The listing builds one solid part. Answer for the finished solid, in the listing's coordinates (mm). Coordinates: 2 decimals unless noted, no trailing zeros. Order: outer loops, then holes, each group sorted by start corner. A loop starts at its lowest first (then second) coordinate and runs counter-clockwise, first axis right, second up. Notation, with made-up numbers: (-22, 10.5) -> (17, 10.5) arc R31 cw to (17, 48.5) -> close; hole circle Ø10 at (20, 10.25). An arc over 180 degrees is marked (long way). Write item = value, one per line. Start each with the question number.
```python
from build123d import *

# Parameters (mm, degrees)
SKETCH3_R                = 76.2
BOSS_EXTRUDE1_DEPTH      = 6.35
BOSS_EXTRUDE1_DEPTH_BACK = 6.35
SKETCH4_R                = 13.0175
SKETCH4_R_2              = 5.953125
CUT_EXTRUDE1_DEPTH       = 13.7


with BuildPart() as part:
    # Sketch3 → Boss-Extrude1 (new body, two sides)
    with BuildSketch(Plane(origin=(0, 0, 0), x_dir=(1, 0, 0), z_dir=(0, 1, 0))) as boss_extrude1_sk:
        Circle(SKETCH3_R)
    extrude(amount=BOSS_EXTRUDE1_DEPTH)
    extrude(boss_extrude1_sk.sketch, amount=-BOSS_EXTRUDE1_DEPTH_BACK)

    # Sketch4 → Cut-Extrude1 (cut, through all)
    with BuildSketch(Plane(origin=(0, 6.35, 0), x_dir=(1, 0, 0), z_dir=(0, 1, 0))):
        Circle(SKETCH4_R)
        with Locations((0, 57.15)):
            Circle(SKETCH4_R_2)
        with Locations((49.493351826, -28.575)):
            Circle(SKETCH4_R_2)
        with Locations((-49.493351826, -28.575)):
            Circle(SKETCH4_R_2)
    extrude(amount=-CUT_EXTRUDE1_DEPTH, mode=Mode.SUBTRACT)


solid = part.part
```
Item 1: Each of these flat-tipped pins is pushed along its axis until it touches: pin 1 (2 mm diameter, centred on y = 2.5, z = 22.5, fed in from +X); pin 2 (15.5 mm diameter, centred on x = 0, z = 0, fed in from -Y); pin 3 (5 mm diameter, centred on x = 10, y = 4.5, fed in from -Z); pin 4 (3 mm diameter, centred on y = 1.5, z = -41.5, fed in from +X). Where does it stop, or does it pass through?
Item 2: Section D-D, the plane z = -57.15 is taken. Give the vertices of the cut face in (x, y), then the cut area to 3 significant figures.
Item 3: For a pull along Z with two mould halves and no side action, classify faces 1 (the flat face through (16, -6.35, -1)), 2 (the cylindrical face through (-46.75, 0.09, 33.86)), 3 (the cylindrical face through (-60.47, 0.089, 46.367)) as pulls with the +Z half, pulls with the -Z half, needs draft (parallel to the pull), parting line crosses it, or undercut.
Item 4: Section C-C, the plane y = 1.5 is taken. Give the number of separate pieces and of enclosed holes in the cut face, then the cut area to 3 significant figures.
Item 5: Consider probe 1 along Z at (x, y) = (0, -1.25); probe 2 along X at (y, z) = (-4, 27); probe 3 along X at (y, z) = (4.75, -53). Determine where each line is inside the solid, lowest interval first.
Item 6: Section A-A, the plane z = 0 is taken. Give the vertices of the cut face in (x, y).
Item 7: Section B-B, the plane x = 0 is taken. Give the vertices of the cut face in (y, z), then the cut area to 3 significant figures.
A:
q1.pin_1 = 73.1
q1.pin_2 = through
q1.pin_3 = -75.83
q1.pin_4 = 64.86
q2.outline = (-50.4, -6.35) -> (-5.95, -6.35) -> (-5.95, 6.35) -> (-50.4, 6.35) -> close; (5.95, -6.35) -> (50.4, -6.35) -> (50.4, 6.35) -> (5.95, 6.35) -> close
q2.area = 1,130 mm^2
q3.face_1 = needs draft
q3.face_2 = undercut
q3.face_3 = parting line crosses it
q4.separate_pieces = 1
q4.enclosed_holes = 4
q4.area = 17,400 mm^2
q5.probe_1 = -76.2 to -63.1, -51.2 to -13.02, 13.02 to 76.2
q5.probe_2 = -71.26 to -55.23, -43.75 to 43.75, 55.23 to 71.26
q5.probe_3 = -54.75 to -4.27, 4.27 to 54.75
q6.outline = (-76.2, -6.35) -> (-13.02, -6.35) -> (-13.02, 6.35) -> (-76.2, 6.35) -> close; (13.02, -6.35) -> (76.2, -6.35) -> (76.2, 6.35) -> (13.02, 6.35) -> close
q7.outline = (-6.35, -76.2) -> (6.35, -76.2) -> (6.35, -63.1) -> (-6.35, -63.1) -> close; (-6.35, -51.2) -> (6.35, -51.2) -> (6.35, -13.02) -> (-6.35, -13.02) -> close; (-6.35, 13.02) -> (6.35, 13.02) -> (6.35, 76.2) -> (-6.35, 76.2) -> close
q7.area = 1,450 mm^2
